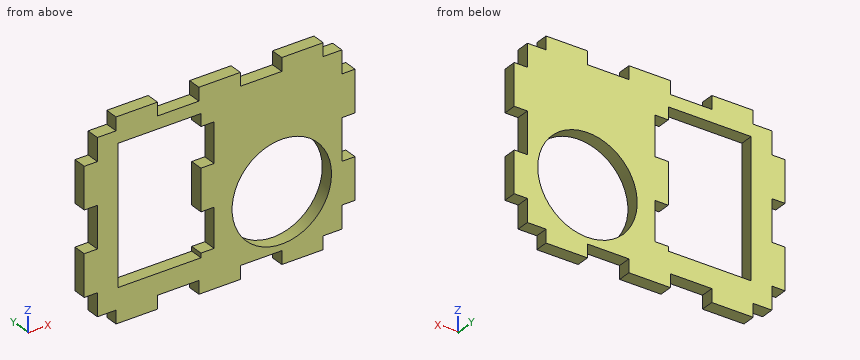
from build123d import *

# Parameters (mm, degrees)
SKETCH1_W           = 65.35
SKETCH1_H           = 47.35
SKETCH1_R           = 12
SKETCH1_W_2         = 20
SKETCH1_H_2         = 33
BOSS_EXTRUDE1_DEPTH = 3.175
SKETCH2_W           = 10
SKETCH2_H           = 3.175
SKETCH2_W_2         = 4.5
SKETCH2_W_3         = 3.175
SKETCH2_H_2         = 10
SKETCH2_H_3         = 5.5
SKETCH2_H_4         = 9.424306971
SKETCH2_H_5         = 9.524418783
CUT_EXTRUDE1_DEPTH  = 3.175


with BuildPart() as part:
    # Sketch1 → Boss-Extrude1 (new body)
    with BuildSketch(Plane(origin=(0, 0, 0), x_dir=(1, 0, 0), z_dir=(0, 1, 0))):
        with Locations((32.675, 23.675)):
            Rectangle(SKETCH1_W, SKETCH1_H)
        with Locations((47.675, 30.675)):
            Circle(SKETCH1_R, mode=Mode.SUBTRACT)
        with Locations((18.175, 22.675)):
            Rectangle(SKETCH1_W_2, SKETCH1_H_2, mode=Mode.SUBTRACT)
    extrude(amount=BOSS_EXTRUDE1_DEPTH)

    # Sketch2 → Cut-Extrude1 (cut)
    with BuildSketch(Plane(origin=(0, 3.175, 0), x_dir=(1, 0, 0), z_dir=(0, 1, 0))):
        with Locations((22.675, 45.7625)):
            Rectangle(SKETCH2_W, SKETCH2_H)
        with Locations((42.675, 45.7625)):
            Rectangle(SKETCH2_W, SKETCH2_H)
        with Locations((59.925, 45.7625)):
            Rectangle(SKETCH2_W_2, SKETCH2_H)
        Polygon((65.35, 47.35), (62.175, 47.35), (62.175, 44.175), (62.175, 38.675), (65.35, 38.675), align=None)
        with Locations((63.7625, 23.675)):
            Rectangle(SKETCH2_W_3, SKETCH2_H_2)
        Polygon((62.175, 3.175), (62.175, 0), (65.35, 0), (65.35, 8.675), (62.175, 8.675), align=None)
        with Locations((59.925, 1.5875)):
            Rectangle(SKETCH2_W_2, SKETCH2_H)
        with Locations((42.675, 1.5875)):
            Rectangle(SKETCH2_W, SKETCH2_H)
        with Locations((22.675, 1.5875)):
            Rectangle(SKETCH2_W, SKETCH2_H)
        with Locations((5.425, 1.5875)):
            Rectangle(SKETCH2_W_2, SKETCH2_H)
        Polygon((3.175, 3.175), (3.175, 8.675), (0, 8.675), (0, 0), (3.175, 0), align=None)
        with Locations((1.5875, 23.675)):
            Rectangle(SKETCH2_W_3, SKETCH2_H_2)
        with Locations((1.5875, 41.425)):
            Rectangle(SKETCH2_W_3, SKETCH2_H_3)
        with Locations((5.425, 45.7625)):
            Rectangle(SKETCH2_W_2, SKETCH2_H)
        with Locations((1.5875, 45.7625)):
            Rectangle(SKETCH2_W_3, SKETCH2_H)
        with Locations((29.7625, 33.387153486)):
            Rectangle(SKETCH2_W_3, SKETCH2_H_4)
        with Locations((29.7625, 13.912790608)):
            Rectangle(SKETCH2_W_3, SKETCH2_H_5)
    extrude(amount=-CUT_EXTRUDE1_DEPTH, mode=Mode.SUBTRACT)


solid = part.part
Can you work these out from the model? Positions are in its coordinate system, mm. Coordinates: 2 decimals unless noted, no trailing zeros. Loops run counter-clockwise (first coordinate to the right, second up) from the corner with the lowest first, then second, coordinate; pieces in that order, holes last. Notation, with made-up numbers: (16, -22) - (48, -22) arc R16 cw to (48, 7) - close; hole circle Ø1 at (70.25, 42). An arc over 180 degrees is marked (long way). Put each result on its own line as item: value. Start each with the question number.
Item 1: For pin 1 (1.6 mm diameter, centred on y = 1.5, z = -32, fed in from -X); pin 2 (1.6 mm diameter, centred on y = 1, z = -5, fed in from +X) (3 decimals); pin 3 (1 mm diameter, centred on y = 1.5, z = -1, fed in from -X) (3 decimals); pin 4 (1.6 mm diameter, centred on y = 2, z = -22, fed in from -X) (3 decimals), each with a flat end and sliding along its axis, tell me the tip position at first contact or that it passes through.
Item 2: Suppose I cut it at A-A (z = -13). Please give me the cut outline in (x, y) (3 decimals), and give its area (3 significant figures).
Item 3: Suppose I cut it at C-C (z = -27.5). Please give me the cut outline in (x, y) (3 decimals), and give its area (3 significant figures).
Item 4: If I drill on line 1 along X through (y, z) = (2.85, -31) (3 decimals); line 2 along X through (y, z) = (2.2, -45) (3 decimals); line 3 along Z through (x, y) = (12.5, 2.2) (3 decimals), over which ranges is the centre line in solid material (lowest first)?
Item 5: Suppose I cut it at B-B (x = 49). Please give me the cut outline in (y, z) (3 decimals), and give its area (3 significant figures).
Item 6: Suppose I cut it at D-D (x = 7). Please give me the cut outline in (y, z) (3 decimals), and give its area (3 significant figures).
Here are the results:
1. pin 1: x = 0
1. pin 2: x = 62.175
1. pin 3: x = 7.675
1. pin 4: x = 3.175
2. outline: (0, 0) - (8.175, 0) - (8.175, 3.175) - (0, 3.175) - close; (31.35, 0) - (65.35, 0) - (65.35, 3.175) - (31.35, 3.175) - close
2. area: 134 mm²
3. outline: (3.175, 0) - (8.175, 0) - (8.175, 3.175) - (3.175, 3.175) - close; (28.175, 0) - (36.103, 0) - (36.103, 3.175) - (28.175, 3.175) - close; (59.247, 0) - (62.175, 0) - (62.175, 3.175) - (59.247, 3.175) - close
3. area: 50.3 mm²
4. line 1: 0 to 8.175, 31.35 to 35.679, 59.671 to 65.35
4. line 2: 7.675 to 17.675, 27.675 to 37.675, 47.675 to 57.675
4. line 3: -47.35 to -39.175, -6.175 to 0
5. outline: (0, -47.35) - (3.175, -47.35) - (3.175, -42.602) - (0, -42.602) - close; (0, -18.748) - (3.175, -18.748) - (3.175, 0) - (0, 0) - close
5. area: 74.6 mm²
6. outline: (0, -44.175) - (3.175, -44.175) - (3.175, -3.175) - (0, -3.175) - close
6. area: 130 mm²
